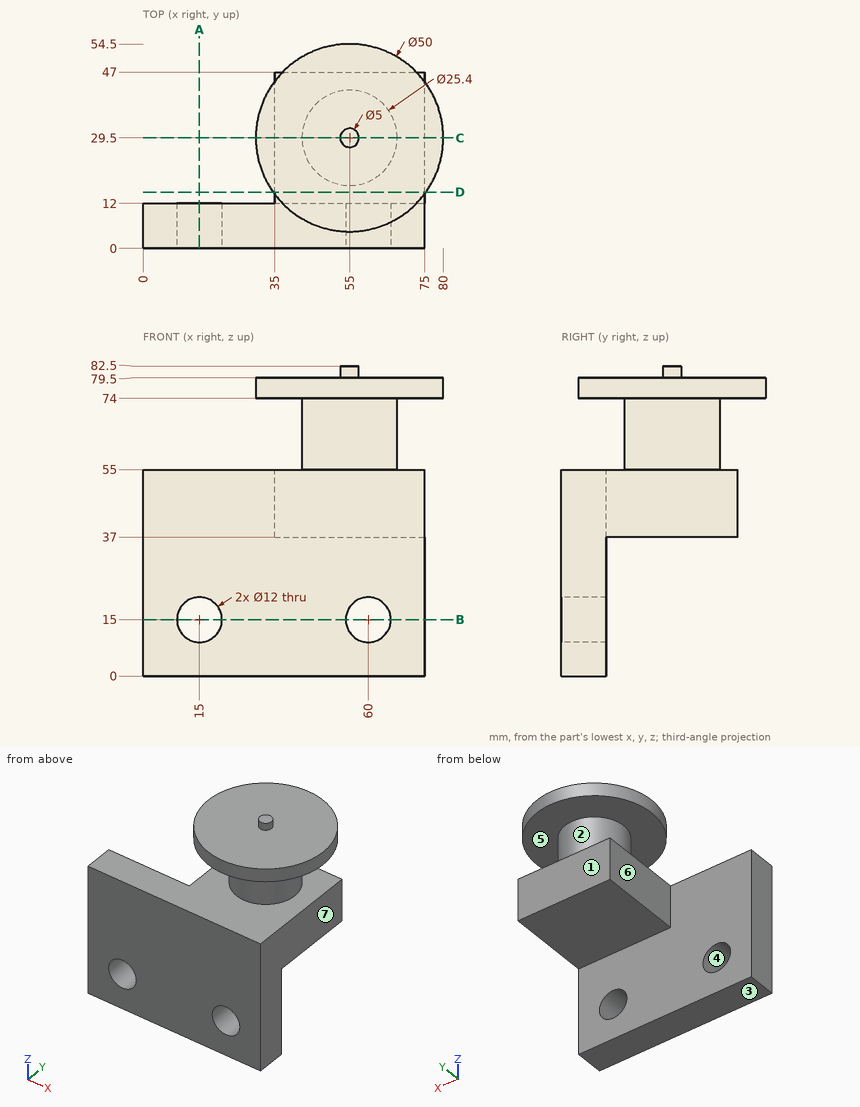
Input: dimensioned drawing with shaded views. Units: mm. Origin: part minimum x, y, z. A direction names the side the tool comes from. Coordinates: 2 decimals unless noted, no trailing zeros. Loops run counter-clockwise (first coordinate to the right, second up) from the corner with the lowest first, then second, coordinate; pieces in that order, holes last. Notation, with made-up numbers: (-27.75, 82.5) - (5.25, 82.5) arc R22 cw to (5.25, 114.5) - close; hole circle Ø9 at (35.5, -25). An arc over 180 degrees is marked (long way). One line per question, with ' | ' between items. Start each with the question number.
(1) Cut plane C-C on y = 29.5. Output: boundary loops of the cut face in (x, z).
(2) Cut plane B-B on z = 15. Output: boundary loops of the cut face in (x, y), and give its area (3 significant figures).
(3) Cut plane A-A on x = 15. Output: boundary loops of the cut face in (y, z), and give its area (3 significant figures).
(4) Reachability of the marked faces 1, 2 and 3 from +Z, -Z, +X, -X, +Y, -Y: full face, straight path, thin tool, end or side. Return the list, or none.
(5) Draft query along X for the marked faces 4, 5, 6 and 7. Return one class per face: +X half, -X half, draft (parallel to the pull), parting line (faces both ways), or undercut.
(6) Cut plane D-D on y = 15. Output: boundary loops of the cut face in (x, z), and give its area (3 significant figures).
(7) Ray query, L1, parallel to Z at x = 60, y = 9; L2, parallel to Z at x = 15, y = 2; L3, parallel to Z at x = 39.5, y = 35. Return the intervals inside material, ascending. Write a range as from..to.
(8) First-contact query: pin 1 (14 mm diameter, centred on y = 25.5, z = 14.5, fed in from +X); pin 2 (1 mm diameter, centred on y = 31, z = 62.5, fed in from +X); pin 3 (8 mm diameter, centred on y = 22.5, z = 58, fed in from -X); pin 4 (2 mm diameter, centred on x = 69.5, y = 22, fed in from +Z). Flat tips, straight axial feed; report the tip coordinate or a pass-through.
Here are the results:
1) outline: (30, 74) - (42.3, 74) - (42.3, 55) - (35, 55) - (35, 37) - (75, 37) - (75, 55) - (67.7, 55) - (67.7, 74) - (80, 74) - (80, 79.5) - (57.5, 79.5) - (57.5, 82.5) - (52.5, 82.5) - (52.5, 79.5) - (30, 79.5) - close
2) outline: (0, 0) - (9, 0) - (9, 12) - (0, 12) - close; (21, 0) - (54, 0) - (54, 12) - (21, 12) - close; (66, 0) - (75, 0) - (75, 12) - (66, 12) - close | area: 612 mm²
3) outline: (0, 0) - (12, 0) - (12, 9) - (0, 9) - close; (0, 21) - (12, 21) - (12, 55) - (0, 55) - close | area: 516 mm²
4) face 1: -Z, +X, -X, +Y | face 2: none | face 3: -Z, +X, -X, +Y, -Y
5) face 4: undercut | face 5: draft | face 6: -X half | face 7: +X half
6) outline: (34.63, 74) - (75.37, 74) - (75.37, 79.5) - (34.63, 79.5) - close; (35, 37) - (75, 37) - (75, 55) - (35, 55) - close | area: 944 mm²
7) L1: 0..9, 21..55, 74..79.5 | L2: 0..9, 21..55 | L3: 37..55, 74..79.5
8) pin 1: through | pin 2: x = 67.66 | pin 3: x = 35 | pin 4: z = 79.5
